Build history of the part. All positions in model axes, mm. A direction names the side the tool comes from. Coordinates: 2 decimals unless noted, no trailing zeros. Order: outer loops, then holes, each group sorted by start corner. A loop starts at its lowest first (then second) coordinate and runs counter-clockwise, first axis right, second up. Notation, with made-up numbers: (12.5, -34) - (20.5, -34) arc R14 ccw to (20.5, -26) - close; hole circle Ø11 at (71, 76.5). An arc over 180 degrees is marked (long way). Write each question's results on one line, items separated by ' | '. Start each with the question number.
from build123d import *

# Parameters (mm, degrees)
SKETCH1_W           = 62.5
SKETCH1_H           = 58
BOSS_EXTRUDE1_DEPTH = 16
FILLET1_R           = 8
SKETCH2_W           = 14
SKETCH2_H           = 52
CUT_EXTRUDE1_DEPTH  = 14
CUT_EXTRUDE2_REACH  = 59.294
SKETCH4_R           = 7.25
BOSS_EXTRUDE3_DEPTH = 24
SKETCH6_R           = 1
BOSS_EXTRUDE5_DEPTH = 2.5


with BuildPart() as part:
    # Sketch1 → Boss-Extrude1 (new body)
    with BuildSketch(Plane(origin=(0, 0, 0), x_dir=(1, 0, 0), z_dir=(0, 1, 0))):
        Rectangle(SKETCH1_W, SKETCH1_H)
    extrude(amount=BOSS_EXTRUDE1_DEPTH)

    # Fillet1
    fillet1_edges = [part.edges().sort_by_distance(p)[0] for p in [
        (-31.25, 16, 0),
        (31.25, 16, 0),
    ]]
    fillet(fillet1_edges, radius=FILLET1_R)

    # Sketch2 → Cut-Extrude1 (cut)
    with BuildSketch(Plane(origin=(0, 16, 0), x_dir=(1, 0, 0), z_dir=(0, 1, 0))):
        Polygon((-29.5, 26), (-15.5, 26), (-15.5, -26), (-29.5, -26), (-29.5, -23.5), (-25.9, -23.5), (-25.9, -8.5), (-29.5, -8.5), (-29.5, 8.5), (-25.9, 8.5), (-25.9, 23.5), (-29.5, 23.5), align=None)
        with Locations((-7.5, 0)):
            Rectangle(SKETCH2_W, SKETCH2_H)
        Polygon((15.5, 26), (29.5, 26), (29.5, 23.5), (25.9, 23.5), (25.9, 8.5), (29.5, 8.5), (29.5, -8.5), (25.9, -8.5), (25.9, -23.5), (29.5, -23.5), (29.5, -26), (15.5, -26), align=None)
        with Locations((7.5, 0)):
            Rectangle(SKETCH2_W, SKETCH2_H)
    extrude(amount=-CUT_EXTRUDE1_DEPTH, mode=Mode.SUBTRACT)

    # Cut-Extrude2: up to this face of the body (flat: up to its plane)
    cut_extrude2_end = Plane(part.part.faces().sort_by_distance((-15.5, 9, 0))[0])
    # Sketch3 → Cut-Extrude2 (cut, up to the picked face)
    with BuildSketch(Plane(origin=(15.5, 0, 0), x_dir=(0, 0, -1), z_dir=(1, 0, 0)), mode=Mode.PRIVATE) as cut_extrude2_sk1:
        Polygon((-26, 16), (-26, 13.5), (-17.5, 8.2), (17.5, 8.2), (26, 13.5), (26, 16), align=None)
    cut_extrude2_tool1 = split(extrude(cut_extrude2_sk1.sketch, amount=-CUT_EXTRUDE2_REACH, mode=Mode.PRIVATE), bisect_by=cut_extrude2_end, keep=Keep.BOTH, mode=Mode.PRIVATE)
    add(cut_extrude2_tool1.solids().sort_by(Axis((15.5, 12.366556, 0), (-1, 0, 0)))[0], mode=Mode.SUBTRACT)

    # Sketch4 → Boss-Extrude3 (add, symmetric)
    with BuildSketch(Plane.XY):
        with Locations((-22.5, 8.75)):
            Circle(SKETCH4_R)
        with Locations((-7.5, 8.75)):
            Circle(SKETCH4_R)
        with Locations((22.5, 8.75)):
            Circle(SKETCH4_R)
        with Locations((7.5, 8.75)):
            Circle(SKETCH4_R)
    extrude(amount=BOSS_EXTRUDE3_DEPTH, both=True)

    # Sketch6 → Boss-Extrude5 (add)
    with BuildSketch(Plane.XY.offset(29)):
        with Locations(Location((-19.25, 2.5, 0), (0, 0, 180))):
            Circle(SKETCH6_R)
        with Locations(Location((-11.25, 2.5, 0), (0, 0, 180))):
            Circle(SKETCH6_R)
    extrude(amount=BOSS_EXTRUDE5_DEPTH)


solid = part.part
Item 1: Slice it at C-C (z = -4). Count the separate pieces of the cut face and the enclosed holes in it, then the cut area to 3 significant figures.
Item 2: Slice it at D-D (x = 21). Write the cut outline in (y, z).
Item 3: Slice it at A-A (x = -7.5). Write the cut outline in (y, z), then the cut area to 3 significant figures.
Item 4: Probe probe 1 along Z at (x, y) = (-3, 9.75); probe 2 along X at (y, z) = (14, 14); probe 3 along Y at (x, z) = (-8, 4). List the from-to ranges inside material, lowest first.
Item 5: Which spindle directions (+Z, -Z, +X, -X, +Y, -Y) get a long thin tool onto all of the face, cutting with end or side? Do faces 3 (the flat face through (-29.5, 4, 0)), 4 (the flat face through (28.2, 13.5, 8.5)). Say none if no direction does.
Item 6: Slice it at B-B (z = -25). Write the cut outline in (x, y), then the cut area to 3 significant figures.
Item 7: Flat gauge pins, fed straight in: P1, Ø1.2, axis at y = 11.5, z = -2, coming from the -X side; P2, Ø1.1, axis at x = 27, y = 12, coming from the +Z side. Where does each tip first touch, or does it go through?
Item 8: Pull direction Z, two halves, no side cores. Call faces 1 (the flat face through (-19, 2, 31.5)), 2 (the flat face through (-28, 3, -23.5)): released by +Z, released by -Z, zero draft, split by the parting line, or undercut.
Resolved:
1) separate pieces: 1 | enclosed holes: 8 | area: 828 mm^2
2) outline: (0, -29) - (16, -29) - (16, -26) - (2, -26) - (2, -24) - (15.84, -24) - (15.84, 24) - (2, 24) - (2, 26) - (16, 26) - (16, 29) - (0, 29) - close
3) outline: (0, -29) - (16, -29) - (16, -26) - (2, -26) - (2, -24) - (16, -24) - (16, 24) - (2, 24) - (2, 26) - (16, 26) - (16, 29) - (0, 29) - close | area: 872 mm^2
4) probe 1: -29 to -26, -24 to 24, 26 to 29 | probe 2: -28.54 to -17.5, -12.5 to -2.5, 2.5 to 12.5, 17.5 to 28.54 | probe 3: 0 to 15.98
5) face 3: none | face 4: +Y
6) outline: (-31.25, 0) - (31.25, 0) - (31.25, 8) arc R8 ccw to (29.5, 12.99) - (29.5, 2) - (15.5, 2) - (15.5, 12.88) - (14.5, 12.88) - (14.5, 2) - (0.5, 2) - (0.5, 12.88) - (-0.5, 12.88) - (-0.5, 2) - (-14.5, 2) - (-14.5, 12.88) - (-15.5, 12.88) - (-15.5, 2) - (-29.5, 2) - (-29.5, 12.99) arc R8 ccw to (-31.25, 8) - close | area: 191 mm^2
7) P1: x = -30.71 | P2: z = 29
8) face 1: released by +Z | face 2: undercut
